Autodesk Inventor part; units mm, degrees
ref_plane "Płaszczyzna konstrukcyjna1" through (13, 18.75, 13) normal (1, 0, 0) x (0, 0, -1)
ref_plane "YZ Plane" through (0, 0, 0) normal (1, 0, 0) x (0, 1, 0)
ref_plane "XZ Plane" through (0, 0, 0) normal (0, 1, 0) x (-1, 0, 0)
sketch "Szkic1" plane through (0, 0, 0) normal (0, 0, 1) x (1, 0, 0)
  circle A0 centre (0, 0) radius 4.25
  line L0 (0, 0) -> (0, 22) construction
  line L1 (-5, 22) -> (5, 22) construction
  line L2 (-5, 17.75) -> (5, 17.75)
  arc A1 (5, 17.75) -> (5, 26.25) centre (5, 22) ccw
  line L3 (5, 26.25) -> (-5, 26.25)
  arc A2 (-5, 26.25) -> (-5, 17.75) centre (-5, 22) ccw
  circle A3 centre (-25, 12) radius 8 construction
  line L4 (-5, 22) -> (-25, 22) construction
  line L5 (-25, 22) -> (-25, 12) construction
  circle A4 centre (-25, 12) radius 2.75
  line L6 (-9.6516, 29.1023) -> (-28.7213, 19.0818)
  arc A5 (-28.7213, 19.0818) -> (-28.3967, 4.7569) centre (-25, 12) ccw
  line L7 (-28.3967, 4.7569) -> (-3.2905, -7.0168)
  arc A6 (-3.2905, -7.0168) -> (6.9098, -3.5096) centre (0, 0) ccw
  line L8 (6.9098, -3.5096) -> (15.9158, 14.2214)
  arc A7 (15.9158, 14.2214) -> (17, 18.75) centre (7, 18.75) ccw
  line L9 (17, 18.75) -> (17, 25.25)
  arc A8 (17, 25.25) -> (12, 30.25) centre (12, 25.25) ccw
  line L10 (12, 30.25) -> (-5, 30.25)
  arc A9 (-5, 30.25) -> (-9.6516, 29.1023) centre (-5, 20.25) ccw
  line L11 (-25, 16.7343) -> (-20.9, 14.3671) construction
  line L12 (-20.9, 14.3671) -> (-20.9, 9.6329) construction
  line L13 (-20.9, 9.6329) -> (-25, 7.2657) construction
  line L14 (-25, 7.2657) -> (-29.1, 9.6329) construction
  line L15 (-29.1, 9.6329) -> (-29.1, 14.3671) construction
  line L16 (-29.1, 14.3671) -> (-25, 16.7343) construction
  line L17 (-5, 22) -> (-5, 30.25) construction
  circle A10 centre (-25, 12) radius 14 construction
  arc A11 (-17.9946, -0.1212) -> (-18.5508, 24.4261) centre (-25, 12) ccw
  dimension "d16" = 28
  dimension "d0" = 8.5
  dimension "d1" = 22
  dimension "d2" = 10
  dimension "d3" = 4.25
  dimension "d4" = 16
  dimension "d5" = 10
  dimension "d6" = 20
  dimension "d7" = 5.5
  dimension "d8" = 12
  dimension "d9" = 4
  dimension "d10" = 7.75
  dimension "d11" = 8.2
  dimension "d12" = 8
  dimension "d13" = 5
  dimension "d14" = 10
  dimension "d15" = 10
extrude "Wyciągnięcie proste1" add sketch "Szkic1" along normal mid plane 26
extrude "Wyciągnięcie proste2" cut sketch "Szkic1" along normal mid plane 16 contours A11 L7 A5 L6
sketch "Szkic2" plane through (0, 0, 13) normal (0, 0, 1) x (1, 0, 0)
  circle A0 centre (-25, 12) radius 2.75
  line L0 (-29.1, 14.3671) -> (-25, 16.7343)
  line L1 (-29.1, 9.6329) -> (-29.1, 14.3671)
  line L2 (-25, 7.2657) -> (-29.1, 9.6329)
  line L3 (-20.9, 9.6329) -> (-25, 7.2657)
  line L4 (-20.9, 14.3671) -> (-20.9, 9.6329)
  line L5 (-25, 16.7343) -> (-20.9, 14.3671)
extrude "Wyciągnięcie proste3" cut sketch "Szkic2" against normal blind 1.5
sketch "Szkic3" plane through (17, 18.75, 13) normal (1, 0, 0) x (0, 0, -1)
  line L0 (26, 6.5) -> (0, 6.5)
  line L1 (0, 0) -> (26, 6.5) construction
  line L2 (0, 6.5) -> (26, 0) construction
  circle A0 centre (13, 3.25) radius 2.25
  line L3 (13, 3.25) -> (13, 11.5) construction
  line L4 (10.9215, 6.85) -> (15.0785, 6.85)
  line L5 (15.0785, 6.85) -> (17.1569, 3.25)
  line L6 (17.1569, 3.25) -> (15.0785, -0.35)
  line L7 (15.0785, -0.35) -> (10.9215, -0.35)
  line L8 (10.9215, -0.35) -> (8.8431, 3.25)
  line L9 (8.8431, 3.25) -> (10.9215, 6.85)
  line L10 (26, 11.5) -> (0, 11.5)
  line L11 (26, 11.5) -> (0, 11.5)
  point P0 (13, -18.75)
  point P1 (13, 6.85)
  dimension "d23" = 4.5
  dimension "d24" = 7.2
ref_plane "Płaszczyzna konstrukcyjna1" through (13, 18.75, 13) normal (1, 0, 0) x (0, 0, -1)
extrude "Wyciągnięcie proste4" cut sketch "Szkic3" against normal up to next contours A0
sketch "Szkic4" plane through (13, 18.75, 13) normal (1, 0, 0) x (0, 0, -1)
  line L0 (10.9215, -0.35) -> (8.8431, 3.25)
  line L1 (15.0785, -0.35) -> (10.9215, -0.35)
  line L2 (17.1569, 3.25) -> (15.0785, -0.35)
  line L3 (15.0785, 6.85) -> (17.1569, 3.25)
  line L4 (10.9215, 6.85) -> (15.0785, 6.85)
  line L5 (8.8431, 3.25) -> (10.9215, 6.85)
  point P0 (13, -18.75)
extrude "Wyciągnięcie proste5" cut sketch "Szkic4" against normal up to surface
properties part number "Y_tensioner"
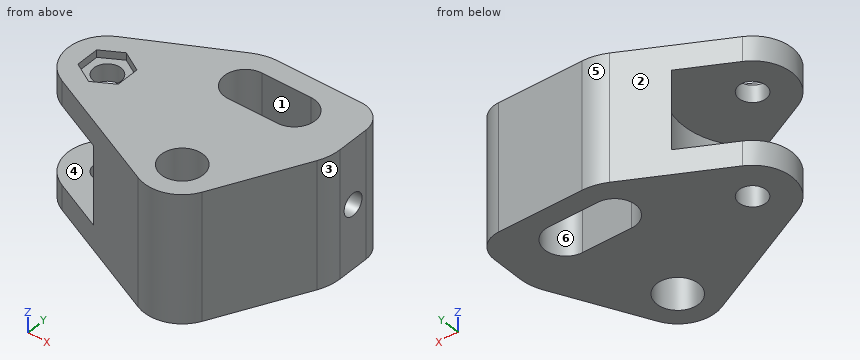
Verification items for the finished model (mm, model axes). Face numbers are marked on the shaded views. A direction names the side the tool comes from. Coordinates: 2 decimals unless noted, no trailing zeros. Write each loop counter-clockwise with the first axis right and the second up, starting at its lowest first coordinate (ties: lowest second). Pieces come first, ordered by that corner, then holes. Notation, with made-up numbers: M -12.75,48 L -6.75,48 A7 ccw -6.75,55 Z; hole C 20.5,-34 d6. An arc over 180 degrees is marked long. Use CSV: the item, a comma, the result in double quotes.
Q1. Mould release check, pull along Y, two halves, no side actions. Record for the marked faces 1, 2 and 3: pulls with the +Y half, pulls with the -Y half, needs draft (parallel to the pull), parting line crosses it, or undercut.
Computed values:
face 1,"undercut"
face 2,"pulls with the +Y half"
face 3,"pulls with the -Y half"
Q2. Section check D-D, the plane z = -5.5. Enter the section's corners in (x, y).
Computed values:
outline,"M -18.55,24.43 A14 cw -17.99,-0.12 L -3.29,-7.02 A7.75 ccw 6.91,-3.51 L 15.92,14.22 A10 ccw 17,18.75 L 17,25.25 A5 ccw 12,30.25 L -5,30.25 A10 ccw -9.65,29.1 Z; hole M -5,17.75 L 5,17.75 A4.25 ccw 5,26.25 L -5,26.25 A4.25 ccw Z; hole C 0,0 d8.5"
Q3. Set-up check for the marked faces 4, 5 and 6: record each of +Z, -Z, +X, -X, +Y, -Y from which the full face is reachable in a straight line by a thin tool's end or side.
Computed values:
face 4,"-X"
face 5,"+Z, -Z, -X, +Y"
face 6,"+Z, -Z"
Q4. Go/stop test with flat-tipped pins: P1, Ø1.6, axis at y = 11, z = 12.5, coming from the -X side; P2, Ø2, axis at x = -15, z = -2.5, coming from the +Y side; P3, Ø10, axis at x = -21.5, z = -6, coming from the -Y side; P4, Ø5, axis at x = -25, y = 12, coming from the +Z side. Record where each tip stops, or that it passes through.
Computed values:
P1,"x = -33"
P2,"y = 26.82"
P3,"y = -0.82"
P4,"through"
Q5. Section check C-C, the plane x = -6. Enter the section's corners in (y, z).
Computed values:
outline,"M -5.75,-13 L 17.87,-13 L 17.87,13 L -5.75,13 Z; M 26.13,-13 L 30.2,-13 L 30.2,13 L 26.13,13 Z"
Q6. Thickness scan on line 1 along Y through (x, z) = (0, 4); line 2 along Z through (x, y) = (-23.5, 17.5); line 3 along Y through (x, z) = (1.5, -11.25). Record the ranges inside material, lowest first. Write a range as [from, to].
Computed values:
line 1,"[-7.75, -4.25], [4.25, 17.75], [26.25, 30.25]"
line 2,"[-13, -8], [8, 13]"
line 3,"[-7.6, -3.98], [3.98, 17.75], [26.25, 30.25]"
Q7. Section check B-B, the plane y = -1. Enter the section's corners in (x, z), and give its area (3 significant figures).
Computed values:
outline,"M -16.12,-13 L -4.13,-13 L -4.13,13 L -16.12,13 Z; M 4.13,-13 L 8.18,-13 L 8.18,13 L 4.13,13 Z"
area,"417 mm²"
Q8. Section check A-A, the plane z = 10.5. Enter the section's corners in (x, y).
Computed values:
outline,"M -28.72,19.08 A8 ccw -28.4,4.76 L -3.29,-7.02 A7.75 ccw 6.91,-3.51 L 15.92,14.22 A10 ccw 17,18.75 L 17,25.25 A5 ccw 12,30.25 L -5,30.25 A10 ccw -9.65,29.1 Z; hole C -25,12 d5.5; hole M -5,17.75 L 5,17.75 A4.25 ccw 5,26.25 L -5,26.25 A4.25 ccw Z; hole C 0,0 d8.5"
